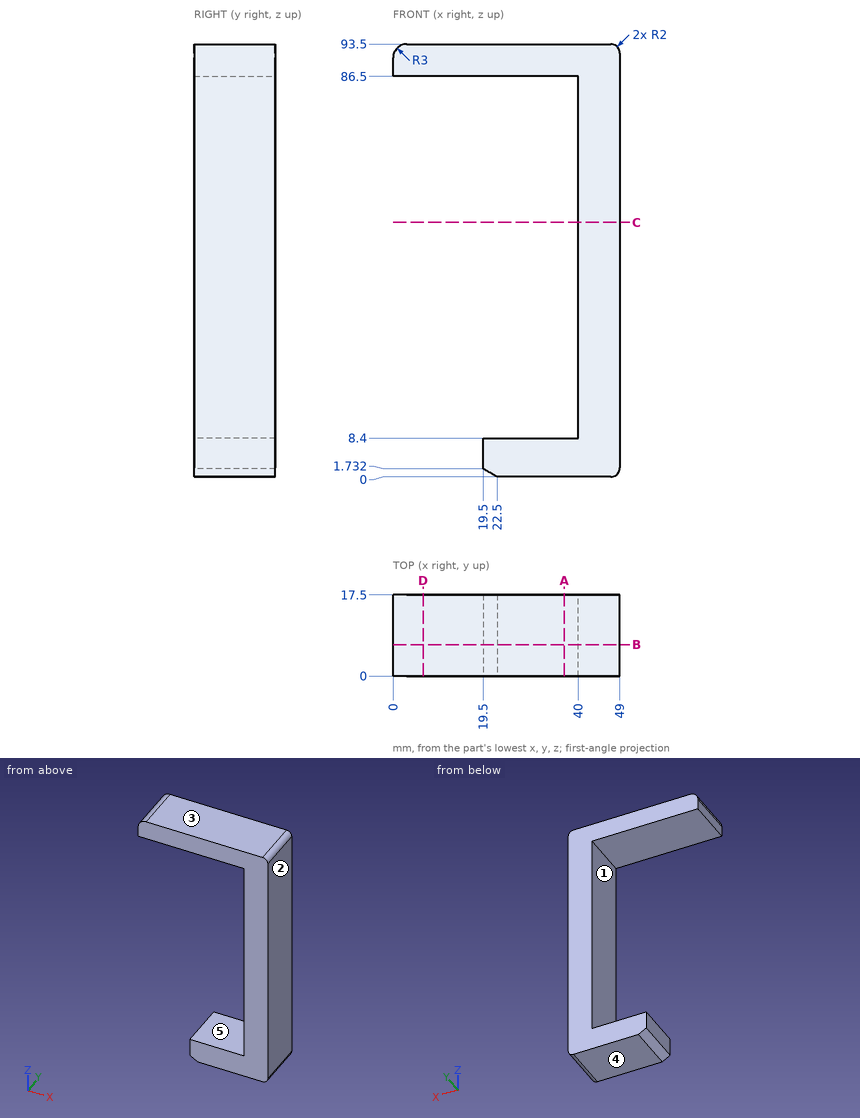
The figure shows three views and two pictorial views of one solid part (mm, origin at its lowest corner). Answer the questions. A direction names the side the tool comes from. Give positions to 0.01 mm unless a question says otherwise; leave off trailing zeros. Loops run counter-clockwise (first coordinate to the right, second up) from the corner with the lowest first, then second, coordinate; pieces in that order, holes last. Notation, with made-up numbers: (-8, -13) -> (49, -13) arc R24 ccw to (49, 17) -> close; hole circle Ø4 at (-2.5, 70.5). An arc over 180 degrees is marked (long way). Put each result on its own line as item: value. Start each with the question number.
Item 1: Which of the six approach directions +Z, -Z, +X, -X, +Y, -Y give full straight-line access (tool end or side, diameter ignored) to the marked faces 4 and 5?
Item 2: The part is cut by section D-D (x = 6.5). Give the vertices of the cut face in (y, z).
Item 3: The part is cut by section B-B (y = 6.75). Give the vertices of the cut face in (x, z), then the cut area to 3 significant figures.
Item 4: Each of these flat-tipped pins is pushed along its axis until it touches: P1, Ø9, axis at y = 9.5, z = 60.5, coming from the -X side; P2, Ø9, axis at x = 11.5, y = 11.5, coming from the -Z side; P3, Ø7.5, axis at y = 9.5, z = 3.5, coming from the -X side. Where does it stop, or does it pass through?
Item 5: Find the intervals of material crossed by L1, parallel to Z at x = 31, y = 5.5; L2, parallel to X at y = 3.25, z = 32; L3, parallel to Z at x = 4.5, y = 13.75, in increasing order. Write a range as [from, to].
Item 6: The part is cut by section A-A (x = 37). Give the vertices of the cut face in (y, z), then the cut area to 4 significant figures.
Item 7: The mould has two halves that part along Z. Classify the marked faces 1, 2 and 3: released by +Z, released by -Z, zero draft, split by the parting line, or undercut.
Item 8: The part is cut by section C-C (z = 55). Give the vertices of the cut face in (x, y), then the cut area to 4 significant figures.
Answers below:
1. face 4: -Z, +X, -X, +Y, -Y
1. face 5: -X, +Y, -Y
2. outline: (0, 86.5) -> (17.5, 86.5) -> (17.5, 93.5) -> (0, 93.5) -> close
3. outline: (0, 86.5) -> (40, 86.5) -> (40, 8.4) -> (19.5, 8.4) -> (19.5, 1.73) -> (22.5, 0) -> (47, 0) arc R2 ccw to (49, 2) -> (49, 91.5) arc R2 ccw to (47, 93.5) -> (3, 93.5) arc R3 ccw to (0, 90.5) -> close
3. area: 1,290 mm2
4. P1: x = 40
4. P2: z = 86.5
4. P3: x = 19.5
5. L1: [0, 8.4], [86.5, 93.5]
5. L2: [40, 49]
5. L3: [86.5, 93.5]
6. outline: (0, 0) -> (17.5, 0) -> (17.5, 8.4) -> (0, 8.4) -> close; (0, 86.5) -> (17.5, 86.5) -> (17.5, 93.5) -> (0, 93.5) -> close
6. area: 269.5 mm2
7. face 1: undercut
7. face 2: zero draft
7. face 3: released by +Z
8. outline: (40, 0) -> (49, 0) -> (49, 17.5) -> (40, 17.5) -> close
8. area: 157.5 mm2
